Here's how the part is built. I have some questions about the finished solid (model axes, mm). Coordinates: 2 decimals unless noted, no trailing zeros. Write each loop counter-clockwise with the first axis right and the second up, starting at its lowest first coordinate (ties: lowest second). Pieces come first, ordered by that corner, then holes. Notation, with made-up numbers: (-9, 67.25) -> (31, 67.25) arc R15 ccw to (31, 71.25) -> close; hole circle Ø10 at (78.25, 76). An arc over 180 degrees is marked (long way). Use a Markdown table: item, result. Add a question column.
```python
from build123d import *

# Parameters (mm, degrees)
F0_W     = 109.854222
F0_H     = 106.995612
F1_DEPTH = 25
F3_D     = 8


with BuildPart() as f1:
    # F0 (on Front) → F1 (new body)
    with BuildSketch(Plane.XZ):
        Rectangle(F0_W, F0_H)
    extrude(amount=F1_DEPTH)

    # F3 (through all)
    with Locations(Plane.XZ.offset(25)):
        with Locations((0, 0)):
            Hole(F3_D / 2)


solid = f1.part
```
Q1. Thinking about a two-plate mould opening in X: for faces 1 (the flat face through (-54.927, -12, -1)), 2 (the flat face through (54.927, -12, -1)), 3 (the flat face through (-1, -12, 53.498)), 4 (the cylindrical face through (0.867, -12.325, -3.905)), which applies, released by +X, released by -X, zero draft, split by the parting line, or undercut?
Q2. Please list where these lines run through material, in increasing order: line 1 (Z direction, x = 0, y = -14.5); line 2 (X direction, y = -22.75, z = 0.5); line 3 (Z direction, x = -1.5, y = -21.5).
Q3. Will this pin go through, and if not, where does the flat tip stop? pin 1 (5 mm diameter, centred on x = 0, z = 0, fed in from -Y).
Q4. Suppose I cut it at B-B, the plane x = 0. Write out the boundary of the cut face in (y, z).
Q5. Suppose I cut it at A-A, the plane z = 0. Write out the boundary of the cut face in (x, y).
Answer key:
| question | item | result |
|---|---|---|
| 1 | face 1 | released by -X |
| 1 | face 2 | released by +X |
| 1 | face 3 | zero draft |
| 1 | face 4 | undercut |
| 2 | line 1 | z = -53.5 to -4, 4 to 53.5 |
| 2 | line 2 | x = -54.93 to -3.97, 3.97 to 54.93 |
| 2 | line 3 | z = -53.5 to -3.71, 3.71 to 53.5 |
| 3 | pin 1 | passes through |
| 4 | outline | (-25, -53.5) -> (0, -53.5) -> (0, -4) -> (-25, -4) -> close; (-25, 4) -> (0, 4) -> (0, 53.5) -> (-25, 53.5) -> close |
| 5 | outline | (-54.93, -25) -> (-4, -25) -> (-4, 0) -> (-54.93, 0) -> close; (4, -25) -> (54.93, -25) -> (54.93, 0) -> (4, 0) -> close |
